For this review, use the dimensioned drawing (mm, ordinates from the lowest corner) and the shaded views. Round coordinates to 2 decimals unless told otherwise and drop trailing zeros. Loops run counter-clockwise (first coordinate to the right, second up) from the corner with the lowest first, then second, coordinate; pieces in that order, holes last. Notation, with made-up numbers: (54.25, 12) -> (87.25, 12) arc R12 ccw to (87.25, 20) -> close; hole circle Ø4 at (21.25, -11.5). An arc over 180 degrees is marked (long way). Answer as CSV lines item,"result". Start each with the question number.
(1) Take a section at C-C, the plane x = 15. Write out the cut boundary in (y, z) (3 decimals).
(2) Take a section at B-B, the plane x = 44.45. Write out the cut boundary in (y, z) (3 decimals), and give its area (3 significant figures).
(3) For P1, Ø4.5, axis at x = 57.15, y = 42.037, coming from the -Z side; P2, Ø1, axis at x = 48.5, z = 25, coming from the +Y side (3 decimals); P3, Ø1, axis at x = 32, z = 83, coming from the +Y side (3 decimals); P4, Ø7, axis at x = 44.45, y = 42.037, coming from the +Z side (3 decimals), all flat-tipped, find the tip position at first contact; note any pin that passes through.
(4) To check wall thickness, follow line 1 (Z direction, x = 58.5, y = 25) (3 decimals); line 2 (Y direction, x = 44.45, z = 2.2) (3 decimals); line 3 (Z direction, x = 14.5, y = 38) (3 decimals). State the ranges of each line that lie inside material, in increasing order. Write a range as from..to.
(5) Take a section at D-D, the plane z = 42. Write out the cut boundary in (x, y) (3 decimals).
(6) Take a section at A-A, the plane y = 11. Write out the cut boundary in (x, z) (3 decimals), and give its area (3 significant figures).
(7) Draft analysis for pull direction Z (two halves, no side actions). For the marked faces 1, 2, 3 and 4, state which applies: +Z half, -Z half, draft (parallel to the pull), parting line (faces both ways), or undercut.
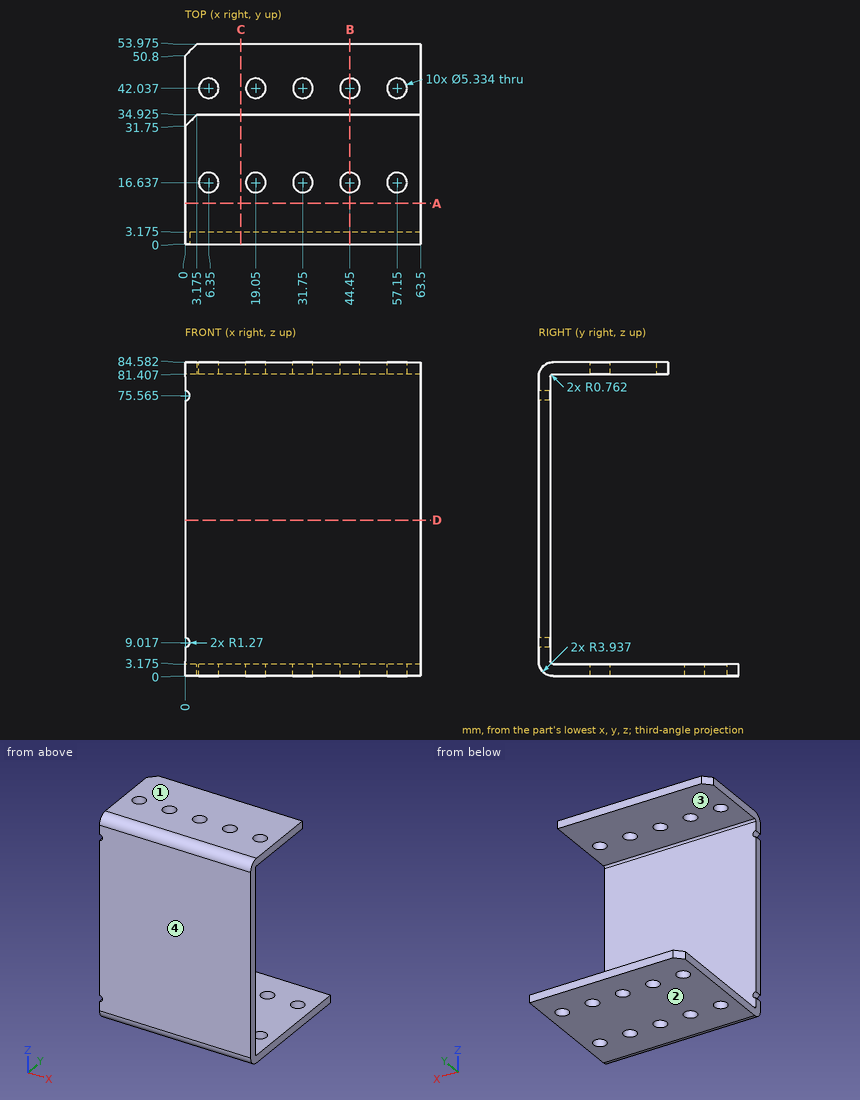
The answers:
1,outline,"(0, 3.937) arc R3.937 ccw to (3.937, 0) -> (53.975, 0) -> (53.975, 3.175) -> (3.937, 3.175) arc R0.762 cw to (3.175, 3.937) -> (3.175, 80.645) arc R0.762 cw to (3.937, 81.407) -> (34.925, 81.407) -> (34.925, 84.582) -> (3.937, 84.582) arc R3.937 ccw to (0, 80.645) -> close"
2,outline,"(0, 3.937) arc R3.937 ccw to (3.937, 0) -> (13.97, 0) -> (13.97, 3.175) -> (3.937, 3.175) arc R0.762 cw to (3.175, 3.937) -> (3.175, 80.645) arc R0.762 cw to (3.937, 81.407) -> (13.97, 81.407) -> (13.97, 84.582) -> (3.937, 84.582) arc R3.937 ccw to (0, 80.645) -> close; (19.304, 0) -> (39.37, 0) -> (39.37, 3.175) -> (19.304, 3.175) -> close; (19.304, 81.407) -> (34.925, 81.407) -> (34.925, 84.582) -> (19.304, 84.582) -> close; (44.704, 0) -> (53.975, 0) -> (53.975, 3.175) -> (44.704, 3.175) -> close"
2,area,"473 mm²"
3,P1,"through"
3,P2,"y = 3.175"
3,P3,"y = 34.925"
3,P4,"z = 3.175"
4,line 1,"0..3.175, 81.407..84.582"
4,line 2,"0.404..13.97, 19.304..39.37, 44.704..53.975"
4,line 3,"0..3.175"
5,outline,"(0, 0) -> (63.5, 0) -> (63.5, 3.175) -> (0, 3.175) -> close"
6,outline,"(0, 0) -> (63.5, 0) -> (63.5, 3.175) -> (0, 3.175) -> close; (0, 81.407) -> (63.5, 81.407) -> (63.5, 84.582) -> (0, 84.582) -> close"
6,area,"403 mm²"
7,face 1,"+Z half"
7,face 2,"-Z half"
7,face 3,"undercut"
7,face 4,"draft"
